from build123d import *

# Parameters (mm, degrees)
SKETCH2_W               = 8
SKETCH2_H               = 20
SKETCH2_W_2             = 11.75
SKETCH2_H_2             = 12.66
BOSS_EXTRUDE1_DEPTH     = 5
SKETCH3_W               = 13.1
SKETCH3_H               = 7
BOSS_EXTRUDE2_DEPTH     = 28
SKETCH4_W               = 5.75
SKETCH4_H               = 12.66
CUT_EXTRUDE1_DEPTH      = 62.587336361
SKETCH5_R               = 2
CUT_EXTRUDE2_DEPTH      = 61.902073035
SKETCH6_R               = 2
CUT_EXTRUDE3_DEPTH      = 60.059292241
SKETCH7_W               = 7
SKETCH7_H               = 28
BOSS_EXTRUDE3_DEPTH     = 19.4
SKETCH8_W               = 27
SKETCH8_H               = 33
BOSS_EXTRUDE4_DEPTH     = 2
SKETCH9_W               = 27
SKETCH9_H               = 33
BOSS_EXTRUDE5_DEPTH     = 2
CUT_EXTRUDE4_DEPTH      = 68.4388612
CUT_EXTRUDE4_DEPTH_BACK = 68.4388612
SKETCH12_W              = 12.66
SKETCH12_H              = 33
CUT_EXTRUDE5_DEPTH      = 63.562468781
SKETCH13_W              = 30
SKETCH13_H              = 7
BOSS_EXTRUDE6_DEPTH     = 33
SKETCH14_R              = 2
CUT_EXTRUDE6_DEPTH      = 88.086164228


with BuildPart() as part:
    # Sketch2 → Boss-Extrude1 (new body)
    with BuildSketch(Plane(origin=(0, 0, 0), x_dir=(1, 0, 0), z_dir=(0, 1, 0))):
        with Locations((-4, 10)):
            Rectangle(SKETCH2_W, SKETCH2_H)
        Polygon((40, 0), (0, 0), (-8, 0), (-8, -7), (3.75, -7), (16.85, -7), (28.6, -7), (48, -7), (48, 0), align=None)
        with Locations((-2.125, -13.33)):
            Rectangle(SKETCH2_W_2, SKETCH2_H_2)
        with Locations((22.725, -13.33)):
            Rectangle(SKETCH2_W_2, SKETCH2_H_2)
        with Locations((44, 10)):
            Rectangle(SKETCH2_W, SKETCH2_H)
    extrude(amount=BOSS_EXTRUDE1_DEPTH)

    # Sketch3 → Boss-Extrude2 (add)
    with BuildSketch(Plane.XZ):
        Polygon((3.75, 19.66), (-8, 19.66), (-8, 0), (0, 0), (3.75, 0), (3.75, 7), align=None)
        with Locations((10.3, 3.5)):
            Rectangle(SKETCH3_W, SKETCH3_H)
        Polygon((16.85, 19.66), (16.85, 7), (16.85, 0), (28.6, 0), (28.6, 7), (28.6, 19.66), align=None)
    extrude(amount=BOSS_EXTRUDE2_DEPTH)

    # Sketch4 → Cut-Extrude1 (cut, through all)
    with BuildSketch(Plane.XZ.offset(28)):
        with Locations((-5.125, 13.33)):
            Rectangle(SKETCH4_W, SKETCH4_H)
        with Locations((25.725, 13.33)):
            Rectangle(SKETCH4_W, SKETCH4_H)
    extrude(amount=-CUT_EXTRUDE1_DEPTH, mode=Mode.SUBTRACT)

    # Sketch5 → Cut-Extrude2 (cut, through all)
    with BuildSketch(Plane.ZY.offset(2.25)):
        with Locations((13.33, -2)):
            Circle(SKETCH5_R)
        with Locations((13.33, -21)):
            Circle(SKETCH5_R)
        with Locations((13.33, -11.5)):
            Circle(SKETCH5_R)
    extrude(amount=-CUT_EXTRUDE2_DEPTH, mode=Mode.SUBTRACT)

    # Sketch6 → Cut-Extrude3 (cut, through all)
    with BuildSketch(Plane.XZ):
        with Locations(Location((43.95, -5, 0), (0, 0, 270))):
            Circle(SKETCH6_R)
        with Locations(Location((43.95, -15, 0), (0, 0, 270))):
            Circle(SKETCH6_R)
        with Locations(Location((-3.95, -5, 0), (0, 0, 270))):
            Circle(SKETCH6_R)
        with Locations(Location((-3.95, -15, 0), (0, 0, 270))):
            Circle(SKETCH6_R)
    extrude(amount=-CUT_EXTRUDE3_DEPTH, mode=Mode.SUBTRACT)

    # Sketch7 → Boss-Extrude3 (add)
    with BuildSketch(Plane(origin=(28.6, 0, 0), x_dir=(0, 0, -1), z_dir=(1, 0, 0))):
        with Locations((-3.5, -14)):
            Rectangle(SKETCH7_W, SKETCH7_H)
    extrude(amount=BOSS_EXTRUDE3_DEPTH)

    # Sketch8 → Boss-Extrude4 (add)
    with BuildSketch(Plane(origin=(48, 0, 0), x_dir=(0, 0, -1), z_dir=(1, 0, 0))):
        with Locations((6.5, -11.5)):
            Rectangle(SKETCH8_W, SKETCH8_H)
    extrude(amount=BOSS_EXTRUDE4_DEPTH)

    # Sketch9 → Boss-Extrude5 (add)
    with BuildSketch(Plane.ZY.offset(8)):
        with Locations((-6.5, -11.5)):
            Rectangle(SKETCH9_W, SKETCH9_H)
    extrude(amount=BOSS_EXTRUDE5_DEPTH)

    # Sketch10 → Cut-Extrude4 (cut, two sides: drawn at the far end of the back side and taken through both)
    with BuildSketch(Plane.ZY.offset(-48).offset(-CUT_EXTRUDE4_DEPTH_BACK)):
        Polygon((-20, 0), (0, -28), (-20, -28), align=None)
    extrude(amount=CUT_EXTRUDE4_DEPTH + CUT_EXTRUDE4_DEPTH_BACK, mode=Mode.SUBTRACT)

    # Sketch12 → Cut-Extrude5 (cut, through all)
    with BuildSketch(Plane.ZY.offset(2.25)):
        with Locations((13.33, -11.5)):
            Rectangle(SKETCH12_W, SKETCH12_H)
    extrude(amount=-CUT_EXTRUDE5_DEPTH, mode=Mode.SUBTRACT)

    # Sketch13 → Boss-Extrude6 (add)
    with BuildSketch(Plane(origin=(0, 5, 0), x_dir=(1, 0, 0), z_dir=(0, 1, 0))):
        with Locations((-25, -3.5)):
            Rectangle(SKETCH13_W, SKETCH13_H)
        with Locations((65, -3.5)):
            Rectangle(SKETCH13_W, SKETCH13_H)
    extrude(amount=-BOSS_EXTRUDE6_DEPTH)

    # Sketch14 → Cut-Extrude6 (cut, through all)
    with BuildSketch(Plane(origin=(0, 0, 0), x_dir=(-1, 0, 0), z_dir=(0, 0, -1))):
        with Locations((35, -23)):
            Circle(SKETCH14_R)
        with Locations((20, -23)):
            Circle(SKETCH14_R)
        with Locations((20, 0)):
            Circle(SKETCH14_R)
        with Locations((35, 0)):
            Circle(SKETCH14_R)
        with Locations((-10, 0)):
            Circle(SKETCH14_R)
        with Locations((-10, -23)):
            Circle(SKETCH14_R)
        with Locations((-30, -23)):
            Circle(SKETCH14_R)
        with Locations((-30, 0)):
            Circle(SKETCH14_R)
        with Locations((-60, 0)):
            Circle(SKETCH14_R)
        with Locations((-60, -23)):
            Circle(SKETCH14_R)
        with Locations((-75, -23)):
            Circle(SKETCH14_R)
        with Locations((-75, 0)):
            Circle(SKETCH14_R)
    extrude(amount=-CUT_EXTRUDE6_DEPTH, mode=Mode.SUBTRACT)


solid = part.part
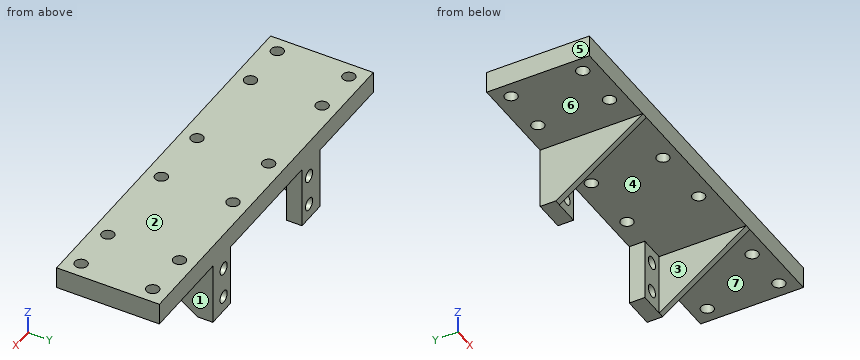
Build history of the part. All positions in model axes, mm. Face numbers are marked on the shaded views. A direction names the side the tool comes from. Coordinates: 2 decimals unless noted, no trailing zeros. Write each loop counter-clockwise with the first axis right and the second up, starting at its lowest first coordinate (ties: lowest second). Pieces come first, ordered by that corner, then holes.
(1) Mould opens along X. For the marked faces 1, 2, 3 and 4 say: pulls with the +X half, pulls with the -X half, needs draft (parallel to the pull), parting line crosses it, or undercut.
(2) Cut at A-A on z = -5. List the corners of the cut face in (x, y), and give its area (3 significant figures).
(3) Cut at C-C on z = 3.25. State how many separate pieces and enclosed holes the cut face has, and give its area (3 significant figures).
(4) 3-axis set-ups, long thin cutter, end or side, ignore diameter. For the marked faces 5, 6 and 7: which of +Z, -Z, +X, -X, +Y, -Y reach the whole face in a straight line?
(5) Cut at B-B on x = -20. List the corners of the cut face in (y, z).
(6) Cut at D-D on x = 43.95. List the corners of the cut face in (y, z), and give its area (3 significant figures).
(7) Drill centre lines: line 1 (Y direction, x = 30, z = 4); line 2 (X direction, y = 1.35, z = -15); line 3 (Y direction, x = 59, z = 0.5). Where is each one in solid material? Low to high.
(8) Pin check, flat tips, straight feed: pin 1 Ø6 at (y, z) = (-12, -5) entering from +X; pin 2 Ø6.5 at (x, y) = (-20, 0) entering from -Z. Stop position of each tip, or through.
Working result:
1. face 1: pulls with the +X half
1. face 2: needs draft
1. face 3: undercut
1. face 4: undercut
2. outline: (-10, -21) - (-8, -21) - (-8, 0) - (-5.95, 0) - (-5.95, 5) - (-10, 5) - close; (-1.95, 0) - (0, 0) - (0, 5) - (-1.95, 5) - close; (40, 0) - (41.95, 0) - (41.95, 5) - (40, 5) - close; (45.95, 0) - (48, 0) - (48, -21) - (50, -21) - (50, 5) - (45.95, 5) - close
2. area: 144 mm2
3. separate pieces: 1
3. enclosed holes: 12
3. area: 3,810 mm2
4. face 5: +Z, -Z, -X, +Y, -Y
4. face 6: -Z, -X, +Y, -Y
4. face 7: -Z, +X, +Y, -Y
5. outline: (-28, 0) - (-25, 0) - (-25, 7) - (-28, 7) - close; (-21, 0) - (-2, 0) - (-2, 7) - (-21, 7) - close; (2, 0) - (5, 0) - (5, 7) - (2, 7) - close
6. outline: (-28, 0) - (0, 0) - (0, -3) - (5, -3) - (5, 7) - (-28, 7) - close; (0, -20) - (5, -20) - (5, -17) - (0, -17) - close; (0, -13) - (5, -13) - (5, -7) - (0, -7) - close
6. area: 291 mm2
7. line 1: y = -28 to -25, -21 to -2, 2 to 5
7. line 2: x = -10 to -5.95, -1.95 to 0, 40 to 41.95, 45.95 to 50
7. line 3: y = -28 to -24.73, -21.27 to -1.73, 1.73 to 5
8. pin 1: stops at x = 50
8. pin 2: stops at z = 0
